Autodesk Inventor part; units mm, degrees
ref_plane "YZ Plane" through (0, 0, 0) normal (1, 0, 0) x (0, 1, 0)
ref_plane "XZ Plane" through (0, 0, 0) normal (0, 1, 0) x (-1, 0, 0)
ref_plane "XY Plane" through (0, 0, 0) normal (0, 0, 1) x (1, 0, 0)
sketch "Sketch1" plane through (0, 0, 0) normal (0, 0, 1) x (1, 0, 0)
  line L0 (0, 0) -> (0, 44.45)
  line L1 (0, 0) -> (44.45, 0)
  line L2 (44.45, 0) -> (44.45, 44.45)
  line L3 (44.45, 44.45) -> (0, 44.45)
  dimension "d1" = 44.45
  dimension "d2" = 44.45
extrude "Extrusion1" add sketch "Sketch1" along normal blind 76.2
sketch "Sketch2" plane through (0, 0, 76.2) normal (0, 0, 1) x (1, 0, 0)
  circle A0 centre (22.225, 22.225) radius 22.225
  line L0 (44.45, 44.45) -> (0, 44.45)
  line L1 (44.45, 0) -> (44.45, 44.45)
  point P0 (0, 0)
  dimension "d5" = 44.45
  dimension "d6" = 22.225
  dimension "d7" = 22.225
extrude "Extrusion2" add sketch "Sketch2" along normal blind 69.85 contours A0
sketch "Sketch3" plane through (0, 0, 0) normal (0, 0, -1) x (-1, 0, 0)
  line L0 (-18.5588, 15.875) -> (-25.8912, 15.875)
  line L1 (-25.8912, 15.875) -> (-29.5573, 22.225)
  line L2 (-29.5573, 22.225) -> (-25.8912, 28.575)
  line L3 (-25.8912, 28.575) -> (-18.5588, 28.575)
  line L4 (-18.5588, 28.575) -> (-14.8927, 22.225)
  line L5 (-14.8927, 22.225) -> (-18.5588, 15.875)
  line L6 (-44.45, 0) -> (0, 0)
  line L7 (0, 0) -> (0, 44.45)
  point P0 (-22.225, 22.225)
  dimension "d10" = 12.7
  dimension "d11" = 22.225
  dimension "d12" = 22.225
extrude "Extrusion3" add sketch "Sketch3" along normal blind 44.45
properties part number "Bag elevator Motor"
Here's how the part is built. I have some questions about the finished solid (model axes, mm). A direction names the side the tool comes from. Coordinates: 2 decimals unless noted, no trailing zeros. Order: outer loops, then holes, each group sorted by start corner. A loop starts at its lowest first (then second) coordinate and runs counter-clockwise, first axis right, second up.
1) Imagine slicing it at B-B on x = 12.5. List the corners of the cut face in (y, z) for me.
2) I need wall thicknesses on line 1 (Z direction, x = 14, y = 10.5); line 2 (Z direction, x = 37, y = 5); line 3 (X direction, y = 21.5, z = 111.5). Which ranges of each line are inside material? Lowest first, please.
3) Which directions (+Z, -Z, +X, -X, +Y, -Y) give clear straight access to the entire face, cutting with the end or side of a thin tool? Please do faces 1 (the face through (40, 5, 76.2)), 2 (the face through (4, 39, 76.2)), 3 (the face through (4, 5, 76.2)), 4 (the face through (39, 40, 76.2)).
4) Imagine slicing it at D-D on x = 20.5. List the corners of the cut face in (y, z) for me (3 decimals), and give its area (3 significant figures).
5) Will these pins go through, and if not, where does the flat tip stop? pin 1 (22 mm diameter, centred on x = 27, y = 13.5, fed in from -Z); pin 2 (4 mm diameter, centred on y = 24.5, z = 120.5, fed in from +X); pin 3 (8 mm diameter, centred on x = 30, y = 6, fed in from -Z); pin 4 (6 mm diameter, centred on x = 24, z = -29.5, fed in from +Y) (3 decimals).
6) Imagine slicing it at C-C on y = 13.5. List the corners of the cut face in (x, z) for me.
7) Imagine slicing it at A-A on z = -14. List the corners of the cut face in (x, y) for me (3 decimals), and give its area (3 significant figures).
Response values:
1. outline: (0, 0) - (44.45, 0) - (44.45, 76.2) - (42.21, 76.2) - (42.21, 146.05) - (2.24, 146.05) - (2.24, 76.2) - (0, 76.2) - close
2. line 1: z = 0 to 146.05
2. line 2: z = 0 to 76.2
2. line 3: x = 0.01 to 44.44
3. face 1: +Z, +X, -Y
3. face 2: +Z, -X, +Y
3. face 3: +Z, -X, -Y
3. face 4: +Z, +X, +Y
4. outline: (0, 0) - (15.875, 0) - (15.875, -44.45) - (28.575, -44.45) - (28.575, 0) - (44.45, 0) - (44.45, 76.2) - (44.383, 76.2) - (44.383, 146.05) - (0.067, 146.05) - (0.067, 76.2) - (0, 76.2) - close
4. area: 7,050 mm2
5. pin 1: stops at z = -44.45
5. pin 2: stops at x = 44.45
5. pin 3: stops at z = 0
5. pin 4: stops at y = 28.575
6. outline: (0, 0) - (44.45, 0) - (44.45, 76.2) - (42.67, 76.2) - (42.67, 146.05) - (1.78, 146.05) - (1.78, 76.2) - (0, 76.2) - close
7. outline: (14.893, 22.225) - (18.559, 15.875) - (25.891, 15.875) - (29.557, 22.225) - (25.891, 28.575) - (18.559, 28.575) - close
7. area: 140 mm2
